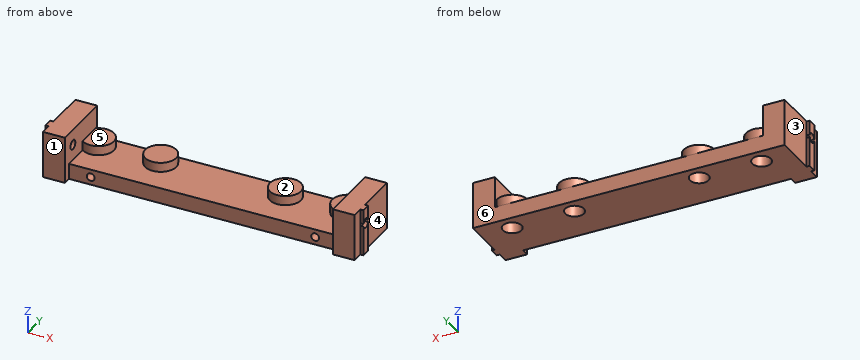
from build123d import *

# Parameters (mm, degrees)
MAIN_DEPTH               = 15
SKETCH2_W                = 86
SKETCH2_H                = 20
TOPEXTRUSION_DEPTH       = 10
SKETCH5_R                = 5
REINFORCEMENTHOLES_DEPTH = 3
SKETCH3_R                = 3
HOLES_DEPTH              = 5
SKETCH4_R                = 1.5
FIXHOLES_DEPTH           = 103
SKETCH6_W                = 86
SKETCH6_H                = 2.5
FORWINDOW_DEPTH          = 6
SKETCH7_R                = 1.25
CUT_EXTRUDE2_DEPTH       = 10


with BuildPart() as part:
    # Sketch1 → Main (new body)
    with BuildSketch(Plane.XY):
        Polygon((-50, 0), (50, 0), (50, 3.55), (51, 3.55), (51, 6.45), (50, 6.45), (50, 20), (-50, 20), (-50, 6.45), (-51, 6.45), (-51, 3.55), (-50, 3.55), align=None)
    extrude(amount=MAIN_DEPTH)

    # Sketch2 → TopExtrusion (cut)
    with BuildSketch(Plane.XY.offset(15)):
        with Locations((0, 10)):
            Rectangle(SKETCH2_W, SKETCH2_H)
    extrude(amount=-TOPEXTRUSION_DEPTH, mode=Mode.SUBTRACT)

    # Sketch5 → ReinforcementHoles (add)
    with BuildSketch(Plane.XY.offset(5)):
        with Locations((-40, 15)):
            Circle(SKETCH5_R)
        with Locations((-20, 15)):
            Circle(SKETCH5_R)
        with Locations((20, 15)):
            Circle(SKETCH5_R)
        with Locations((40, 15)):
            Circle(SKETCH5_R)
    extrude(amount=REINFORCEMENTHOLES_DEPTH)

    # Sketch3 → Holes (cut)
    with BuildSketch(Plane.XY):
        with Locations((-40, 15)):
            Circle(SKETCH3_R)
        with Locations((20, 15)):
            Circle(SKETCH3_R)
    holes = extrude(amount=HOLES_DEPTH, mode=Mode.SUBTRACT)

    # Mirror1: Holes across plane
    add(holes.mirror(Plane(origin=(0, 0, 0), x_dir=(0, 0, 1), z_dir=(1, 0, 0))), mode=Mode.SUBTRACT)

    # Sketch4 → FixHoles (cut, through all)
    with BuildSketch(Plane(origin=(51, 0, 0), x_dir=(0, 0, -1), z_dir=(1, 0, 0))):
        with Locations((-10, 5)):
            Circle(SKETCH4_R)
    extrude(amount=-FIXHOLES_DEPTH, mode=Mode.SUBTRACT)

    # Sketch6 → ForWindow (cut, through all)
    with BuildSketch(Plane.XY.offset(5)):
        with Locations((0, 1.25)):
            Rectangle(SKETCH6_W, SKETCH6_H)
    extrude(amount=-FORWINDOW_DEPTH, mode=Mode.SUBTRACT)

    # Sketch7 → Cut-Extrude2 (cut)
    with BuildSketch(Plane(origin=(0, 2.5, 0), x_dir=(-1, 0, 0), z_dir=(0, -1, 0))):
        with Locations((36, -2.5)):
            Circle(SKETCH7_R)
        with Locations((-36, -2.5)):
            Circle(SKETCH7_R)
    extrude(amount=-CUT_EXTRUDE2_DEPTH, mode=Mode.SUBTRACT)


solid = part.part
CAD build for the part. Positions are in the model's coordinates, mm. Face numbers are marked on the shaded views. A direction names the side the tool comes from. Give positions to 0.01 mm unless a question says otherwise; leave off trailing zeros. Write each loop counter-clockwise with the first axis right and the second up, starting at its lowest first coordinate (ties: lowest second). Pieces come first, ordered by that corner, then holes. Notation, with made-up numbers: (39.5, 37) -> (75.5, 37) arc R16 cw to (75.5, 57) -> close; hole circle Ø5 at (45, -20.5). An arc over 180 degrees is marked (long way). Return JSON: item names as keys, results as strings.
Item 1: Band-saw the part on D-D (x = 39). List the corners of the cut face in (y, z).
Answer below:
{"outline": "(2.5, 0) -> (12.17, 0) -> (12.17, 5) -> (17.83, 5) -> (17.83, 0) -> (20, 0) -> (20, 5) -> (19.9, 5) -> (19.9, 8) -> (10.1, 8) -> (10.1, 5) -> (2.5, 5) -> close"}
Item 2: Band-saw the part on B-B (z = 2.5). List the corners of the cut face in (x, y).
Answer below:
{"outline": "(-51, 3.55) -> (-50, 3.55) -> (-50, 0) -> (-43, 0) -> (-43, 2.5) -> (-37.25, 2.5) -> (-37.25, 12.5) -> (-34.75, 12.5) -> (-34.75, 2.5) -> (34.75, 2.5) -> (34.75, 12.5) -> (37.25, 12.5) -> (37.25, 2.5) -> (43, 2.5) -> (43, 0) -> (50, 0) -> (50, 3.55) -> (51, 3.55) -> (51, 6.45) -> (50, 6.45) -> (50, 20) -> (-50, 20) -> (-50, 6.45) -> (-51, 6.45) -> close; hole circle Ø6 at (-40, 15); hole circle Ø6 at (-20, 15); hole circle Ø6 at (20, 15); hole circle Ø6 at (40, 15)"}
Item 3: Drill centre lines: probe 1 along X at (y, z) = (6, 2.5); probe 2 along X at (y, z) = (7.5, 2.5); probe 3 along X at (y, z) = (15.75, 6.75). Where is each one in solid material? Low to high.
Answer below:
{"probe 1": "x = -51 to -37.25, -34.75 to 34.75, 37.25 to 51", "probe 2": "x = -50 to -37.25, -34.75 to 34.75, 37.25 to 50", "probe 3": "x = -50 to -35.06, -24.94 to -15.06, 15.06 to 24.94, 35.06 to 50"}
Item 4: Drop flat-ended pins along their axis: pin 1 (1.8 mm diameter, centred on y = 2.5, z = 6.5, fed in from -X); pin 2 (8 mm diameter, centred on x = -19, y = 15, fed in from +Z); pin 3 (7 mm diameter, centred on x = 20, y = 15, fed in from -Z); pin 4 (5 mm diameter, centred on x = -11.5, y = 2.5, fed in from +Z). Give the stop position or say it passes through.
Answer below:
{"pin 1": "stops at x = -50", "pin 2": "stops at z = 8", "pin 3": "stops at z = 0", "pin 4": "stops at z = 5"}
Item 5: Tool access for the marked faces 1, 2 and 3: list every direction of +Z, -Z, +X, -X, +Y, -Y with a clear straight run to the whole face (end or side of a thin tool).
Answer below:
{"face 1": "+Z, -Z, +X, -X, -Y", "face 2": "+Z, +Y, -Y", "face 3": "+Z, -Z, -X, +Y"}
Item 6: Band-saw the part on A-A (y = 5). List the corners of the cut face in (x, z), then the cut area to 3 significant figures.
Answer below:
{"outline": "(-51, 0) -> (51, 0) -> (51, 8.5) -> (43, 8.5) -> (43, 5) -> (-43, 5) -> (-43, 8.5) -> (-51, 8.5) -> close; (-51, 11.5) -> (-43, 11.5) -> (-43, 15) -> (-51, 15) -> close; (43, 11.5) -> (51, 11.5) -> (51, 15) -> (43, 15) -> close; hole circle Ø2.5 at (-36, 2.5); hole circle Ø2.5 at (36, 2.5)", "area": "612 mm2"}
Item 7: Band-saw the part on C-C (x = -36). List the corners of the cut face in (y, z).
Answer below:
{"outline": "(2.5, 0) -> (20, 0) -> (20, 5) -> (18, 5) -> (18, 8) -> (12, 8) -> (12, 5) -> (2.5, 5) -> (2.5, 3.75) -> (12.5, 3.75) -> (12.5, 1.25) -> (2.5, 1.25) -> close"}
Item 8: Two-plate mould, pull along X, no slides. Class the marked faces 4, 5 and 6: +X half, -X half, draft (parallel to the pull), parting line (faces both ways), or undercut.
Answer below:
{"face 4": "+X half", "face 5": "undercut", "face 6": "draft"}
